CAD build for the part. Positions are in the model's coordinates, mm. A direction names the side the tool comes from. Give positions to 0.01 mm unless a question says otherwise; leave off trailing zeros. Loops run counter-clockwise (first coordinate to the right, second up) from the corner with the lowest first, then second, coordinate; pieces in that order, holes last. Notation, with made-up numbers: M 77,27.5 L 100,27.5 A30 cw 100,52.5 Z; hole C -15.5,-14.75 d10. An arc over 180 degrees is marked long. One line per question, with ' | ' between items.
```python
from build123d import *

# Parameters (mm, degrees)
F0_W     = 80
F0_H     = 60
F1_DEPTH = 25
F3_DEPTH = 2
F4_W     = 80
F4_H     = 25
F5_DEPTH = 16
F6_R     = 4
F7_DEPTH = 4
F9_D     = 4.2
F10_SIZE = 0.5


with BuildPart() as f1:
    # F0 (on Top) → F1 (new body)
    with BuildSketch(Plane.XY):
        Rectangle(F0_W, F0_H)
    extrude(amount=F1_DEPTH)

    # F2 (on face) → F3 (cut)
    with BuildSketch(Plane(origin=(0, 0, 0), x_dir=(1, 0, 0), z_dir=(0, 0, -1))):
        Polygon((30, 10), (30, 20), (-30, 20), (-30, 10), (-40, 10), (-40, -10), (-30, -10), (-30, -20), (30, -20), (30, -10), (40, -10), (40, 10), align=None)
    extrude(amount=-F3_DEPTH, mode=Mode.SUBTRACT)

    # F4 (on face) → F5 (cut)
    with BuildSketch(Plane.XY.offset(25)):
        Rectangle(F4_W, F4_H)
    extrude(amount=-F5_DEPTH, mode=Mode.SUBTRACT)

    # F6 (on face) → F7 (cut)
    with BuildSketch(Plane.XY.offset(9)):
        with Locations((-32, 0)):
            Circle(F6_R)
    extrude(amount=-F7_DEPTH, mode=Mode.SUBTRACT)

    # F9 (through all)
    with Locations(Plane.XZ.offset(30)):
        with Locations((-16, 19)):
            Hole(F9_D / 2)

    # F10
    f10_edges = [f1.edges().sort_by_distance(p)[0] for p in [
        (35, 10, 0),
        (30, 15, 0),
        (0, 20, 0),
        (-30, 15, 0),
        (-35, 10, 0),
        (-40, 20, 0),
        (0, 30, 0),
        (40, 20, 0),
        (0, -30, 0),
        (-40, -20, 0),
        (-35, -10, 0),
        (-30, -15, 0),
        (0, -20, 0),
        (30, -15, 0),
        (35, -10, 0),
        (40, -20, 0),
        (-40, 10, 1),
        (-40, 0, 2),
        (-40, -10, 1),
        (-40, -30, 12.5),
        (-40, -21.25, 25),
        (-40, -12.5, 17),
        (-40, 0, 9),
        (-40, 12.5, 17),
        (-40, 21.25, 25),
        (-40, 30, 12.5),
        (0, -30, 25),
        (40, -30, 12.5),
        (-18.1, -30, 19),
        (40, -10, 1),
        (40, 0, 2),
        (40, 10, 1),
        (40, 30, 12.5),
        (40, 21.25, 25),
        (40, 12.5, 17),
        (40, 0, 9),
        (40, -12.5, 17),
        (40, -21.25, 25),
        (0, 30, 25),
        (-18.1, 30, 19),
    ]]
    chamfer(f10_edges, length=F10_SIZE)


solid = f1.part
```
Item 1: Saw through at C-C on y = 18. Give the cut face in (x, z).
Conclusion:
outline: M -40,0.5 L -39.5,0 L -30.5,0 L -30,0.5 L -30,2 L 30,2 L 30,0.5 L 30.5,0 L 39.5,0 L 40,0.5 L 40,24.5 L 39.5,25 L -39.5,25 L -40,24.5 Z; hole C -16,19 d4.2
Item 2: Saw through at A-A on z = 19. Give the cut face in (x, y), and give its area (3 significant figures).
Conclusion:
outline: M -40,-29.5 L -39.5,-30 L -18.6,-30 L -18.1,-29.5 L -18.1,-12.5 L -39.5,-12.5 L -40,-13 Z; M -40,13 L -39.5,12.5 L -18.1,12.5 L -18.1,29.5 L -18.6,30 L -39.5,30 L -40,29.5 Z; M -13.9,-29.5 L -13.4,-30 L 39.5,-30 L 40,-29.5 L 40,-13 L 39.5,-12.5 L -13.9,-12.5 Z; M -13.9,12.5 L 39.5,12.5 L 40,13 L 40,29.5 L 39.5,30 L -13.4,30 L -13.9,29.5 Z | area: 2,650 mm²
Item 3: Saw through at B-B on x = -16. State how many separate pieces and enclosed holes the cut face has, and give its area (3 significant figures).
Conclusion:
separate pieces: 3 | enclosed holes: 0 | area: 872 mm²
Item 4: 3-axis set-ups, long thin cutter, end or side, ignore diameter. For faces 1 (the flat face through (-32, 0, 5)), 2 (the flat face through (-1, -24, 0)), 3 (the flat face through (-1, -12.5, 17)): which of +Z, -Z, +X, -X, +Y, -Y reach the whole face in a straight line?
Conclusion:
face 1: +Z | face 2: -Z, +X, -X, +Y, -Y | face 3: +Z, +X, -X
Item 5: Mould opens along Y. For faces 4 (the cylindrical face through (-35.2, -2.4, 7)), 5 (the flat face through (-1, 30, 12)), 6 (the flat face through (-1, -30, 12)), 7 (the flat face through (40, 0, 7)) say: pulls with the +Y half, pulls with the -Y half, needs draft (parallel to the pull), parting line crosses it, or undercut.
Conclusion:
face 4: undercut | face 5: pulls with the +Y half | face 6: pulls with the -Y half | face 7: needs draft
Item 6: Drill centre lines: line 1 along Y through (x, z) = (-2, 23.25); line 2 along Z through (x, y) = (-16, 17); line 3 along Z through (x, y) = (-16, 21). Where is each one in solid material? Low to high. Write a range as [from, to].
Conclusion:
line 1: [-30, -12.5], [12.5, 30] | line 2: [2, 16.9], [21.1, 25] | line 3: [0, 16.9], [21.1, 25]
Item 7: Drop flat-ended pins along their axis: P1, Ø9, axis at x = -33, y = 1, coming from the +Z side; P2, Ø20, axis at x = -19, y = -8.5, coming from the -Z side; P3, Ø6.5, axis at x = -16, z = 19, coming from the -Y side. Give the stop position or say it passes through.
Conclusion:
P1: z = 9 | P2: z = 2 | P3: y = -30
Item 8: Saw through at D-D on z = 13.25. Give the cut face in (x, y).
Conclusion:
outline: M -40,-29.5 L -39.5,-30 L 39.5,-30 L 40,-29.5 L 40,-13 L 39.5,-12.5 L -39.5,-12.5 L -40,-13 Z; M -40,13 L -39.5,12.5 L 39.5,12.5 L 40,13 L 40,29.5 L 39.5,30 L -39.5,30 L -40,29.5 Z
